Verification items for the finished model (mm, model axes). Give positions to 0.01 mm unless a question says otherwise; leave off trailing zeros. Loops run counter-clockwise (first coordinate to the right, second up) from the corner with the lowest first, then second, coordinate; pieces in that order, holes last. Notation, with made-up numbers: (15.25, 83.25) - (23.25, 83.25) arc R16 cw to (23.25, 100.25) - close; hole circle Ø8 at (13, 19.25). An arc over 180 degrees is marked (long way). One line per item, written item: value. Start each with the question number.
1. Sectioned sample at D-D (z = -815). Record the cut outline in (x, y), plus the area to 3 significant figures.
2. Gauge pin test, flat ends, axial feed: pin 1 (12 mm diameter, centred on y = 18.5, z = 443, fed in from +X); pin 2 (10 mm diameter, centred on y = 20.5, z = 384, fed in from +X). Record the tip position at first contact, or that the pin passes through.
3. Scan lines: L1, parallel to X at y = 9.5, z = 0; L2, parallel to X at y = 4.5, z = 319.5; L3, parallel to Z at x = -314, y = 19. Record each from-to range of solid material in increasing order. Write a range as [from, to].
4. Sectioned sample at A-A (z = 0). Record the cut outline in (x, y).
5. Sectioned sample at B-B (x = 0). Record the cut outline in (y, z).
6. Mould release check, pull along X, two halves, no side actions. Record for faces 1 (the flat face through (513.37, 12.32, -891.64)), 2 (the flat face through (700, 25, -221)), 3 (the cylindrical face through (-213.526, 12.325, -678.045)): pulls with the +X half, pulls with the -X half, needs draft (parallel to the pull), parting line crosses it, or undercut.
7. Sectioned sample at C-C (y = 17.5). Record the cut outline in (x, z), plus the area to 3 significant figures.
from build123d import *

# Parameters (mm, degrees)
BOSS_EXTRUDE1_DEPTH = 25
CUT_EXTRUDE4_REACH  = 1392.455
SKETCH2_R           = 710.8712965


with BuildPart() as part:
    # Sketch1 → Boss-Extrude1 (new body)
    with BuildSketch(Plane(origin=(0, 0, 0), x_dir=(1, 0, 0), z_dir=(0, 1, 0))):
        Polygon((438.317943801, 934.970880832), (590.549562699, 847.079914683), (1028.8675065, 87.89096615), (1028.8675065, -87.89096615), (590.549562699, -847.079914683), (438.317943801, -934.970880832), (-438.317943801, -934.970880832), (-590.549562699, -847.079914683), (-1028.8675065, -87.89096615), (-1028.8675065, 87.89096615), (-590.549562699, 847.079914683), (-438.317943801, 934.970880832), align=None)
    extrude(amount=BOSS_EXTRUDE1_DEPTH)

    # Sketch2 → Cut-Extrude4 (cut, up to next)
    with BuildSketch(Plane(origin=(0, 0, 0), x_dir=(1, 0, 0), z_dir=(0, 1, 0)), mode=Mode.PRIVATE) as cut_extrude4_sk1:
        with Locations(Location((0, 0, 0), (0, 0, 90))):
            Circle(SKETCH2_R)
    cut_extrude4_tool1 = extrude(cut_extrude4_sk1.sketch, amount=CUT_EXTRUDE4_REACH, mode=Mode.PRIVATE) & part.part
    add(cut_extrude4_tool1.solids().sort_by_distance((0, 0, 0))[0], mode=Mode.SUBTRACT)


solid = part.part
Results are:
1. outline: (-609.07, 0) - (609.07, 0) - (609.07, 25) - (-609.07, 25) - close
1. area: 30,500 mm^2
2. pin 1: stops at x = 827.31
2. pin 2: stops at x = 860.8
3. L1: x = [-1028.87, -710.87], [710.87, 1028.87]
3. L2: x = [-895.15, -635.03], [635.03, 895.15]
3. L3: z = [-934.97, -637.76], [637.76, 934.97]
4. outline: (-1028.87, 0) - (-710.87, 0) - (-710.87, 25) - (-1028.87, 25) - close; (710.87, 0) - (1028.87, 0) - (1028.87, 25) - (710.87, 25) - close
5. outline: (0, -934.97) - (25, -934.97) - (25, -710.87) - (0, -710.87) - close; (0, 710.87) - (25, 710.87) - (25, 934.97) - (0, 934.97) - close
6. face 1: pulls with the +X half
6. face 2: needs draft
6. face 3: undercut
7. outline: (-1028.87, -87.89) - (-590.55, -847.08) - (-438.32, -934.97) - (438.32, -934.97) - (590.55, -847.08) - (1028.87, -87.89) - (1028.87, 87.89) - (590.55, 847.08) - (438.32, 934.97) - (-438.32, 934.97) - (-590.55, 847.08) - (-1028.87, 87.89) - close; hole circle Ø1421.74 at (0, 0)
7. area: 1,410,000 mm^2
